Build history of the part. All positions in model axes, mm. A direction names the side the tool comes from. Coordinates: 2 decimals unless noted, no trailing zeros. Write each loop counter-clockwise with the first axis right and the second up, starting at its lowest first coordinate (ties: lowest second). Pieces come first, ordered by that corner, then holes. Notation, with made-up numbers: M 30,87.5 L 46,87.5 A27 cw 46,120.5 Z; hole C 59.5,-38.75 d4. An arc over 180 degrees is marked long. Use CSV: the item, a comma, the result in double quotes. Start each with the question number.
```python
from build123d import *

# Parameters (mm, degrees)
SKETCH1_R           = 2
BOSS_EXTRUDE1_DEPTH = 5
FILLET1_R           = 2


with BuildPart() as part:
    # Sketch1 → Boss-Extrude1 (new body)
    # profile 1 of 4: a face of its own
    with BuildSketch(Plane.XY):
        Polygon((8, 4), (-8, 4), (-8, 2.7), (-8, 0), (-8, -4), (8, -4), align=None)
        with Locations((-4, 0)):
            Circle(SKETCH1_R, mode=Mode.SUBTRACT)
        with BuildLine():
            ThreePointArc((6, 0), (4, -2), (2, 0))
            ThreePointArc((2, 0), (4, 2), (6, 0))
        make_face(mode=Mode.SUBTRACT)
    # profile 2 of 4: a face of its own
    with BuildSketch(Plane.XY):
        with BuildLine():
            Line((-8, 2.7), (-8, 4))
            Line((-8, 4), (-13.191868154, 4))
            ThreePointArc((-13.191868154, 4), (-13.048225449, 3.357041359), (-13, 2.7))
            Line((-13, 2.7), (-8, 2.7))
        make_face()
    # profile 3 of 4: a face of its own
    with BuildSketch(Plane.XY):
        with BuildLine():
            Line((-8, 0), (-8, 2.7))
            Line((-8, 2.7), (-13, 2.7))
            ThreePointArc((-13, 2.7), (-13.230925159, 1.276975053), (-13.9, 0))
            Line((-13.9, 0), (-8, 0))
        make_face()
    # profile 4 of 4: a face of its own
    with BuildSketch(Plane.XY):
        with BuildLine():
            ThreePointArc((-13, 2.7), (-13.048225449, 3.357041359), (-13.191868154, 4))
            ThreePointArc((-13.191868154, 4), (-21.931098884, 3.484450558), (-13.9, 0))
            ThreePointArc((-13.9, 0), (-13.230925159, 1.276975053), (-13, 2.7))
        make_face()
        with BuildLine():
            ThreePointArc((-20, 2.7), (-17.5, 5.2), (-15, 2.7))
            ThreePointArc((-15, 2.7), (-17.5, 0.2), (-20, 2.7))
        make_face(mode=Mode.SUBTRACT)
    extrude(amount=BOSS_EXTRUDE1_DEPTH)

    # Fillet1
    fillet1_edges = [part.edges().sort_by_distance(p)[0] for p in [
        (-8, 0, 2.5),
        (-13.9, 0, 2.5),
        (-13.191868154, 4, 2.5),
    ]]
    fillet(fillet1_edges, radius=FILLET1_R)


solid = part.part
```
1. Pull direction X, two halves, no side cores. Call faces 4 (the cylindrical face through (-13.764, -0.148, 2.535)), 5 (the flat face through (-7, 0, 0)), 6 (the flat face through (-8, -3, 2)): pulls with the +X half, pulls with the -X half, needs draft (parallel to the pull), parting line crosses it, or undercut.
2. Slice it at C-C (y = 2.7). List the corners of the cut face in (x, z), and give its area (3 significant figures).
3. 3-axis set-ups, long thin cutter, end or side, ignore diameter. For faces 1 (the flat face through (-2, 4, 2)), 2 (the cylindrical face through (-8.57, -0.6, 2.54)), 3 (the cylindrical face through (-21.933, 3.472, 2.465)): which of +Z, -Z, +X, -X, +Y, -Y reach the whole face in a straight line?
4. Slice it at D-D (y = 0.75). List the corners of the cut face in (x, z).
5. Slice it at B-B (z = 4.1). List the corners of the cut face in (x, y).
6. Drill centre lines: line 1 along Y through (x, z) = (4, 1.3); line 2 along Y through (x, z) = (-17.5, 1.2); line 3 along X through (y, z) = (-1.25, 3.55). Where is each one in solid material? Low to high. Write a range as from..to.
7. Slice it at A-A (x = 4). List the corners of the cut face in (y, z), and give its area (3 significant figures).
8. Flat gauge pins, fed straight in: pin 1 (3 mm diameter, centred on y = 0, z = 1, fed in from -X); pin 2 (1.5 mm diameter, centred on y = 3.5, z = 3, fed in from -X); pin 3 (2 mm diameter, centred on x = -12.5, z = 1.5, fed in from +Y); pin 4 (2.5 mm diameter, centred on x = -4, z = 3, fed in from +Y). Where does each tip first touch, or does it go through?
Established:
1,face 4,"undercut"
1,face 5,"needs draft"
1,face 6,"pulls with the -X half"
2,outline,"M -22,0 L -20,0 L -20,5 L -22,5 Z; M -15,0 L 8,0 L 8,5 L -15,5 Z"
2,area,"125 mm2"
3,face 1,"+Z, -Z, +X, +Y"
3,face 2,"+Z, -Z, -Y"
3,face 3,"+Z, -Z"
4,outline,"M -21.56,0 L -19.06,0 L -19.06,5 L -21.56,5 Z; M -15.94,0 L -5.85,0 L -5.85,5 L -15.94,5 Z; M -2.15,0 L 2.15,0 L 2.15,5 L -2.15,5 Z; M 5.85,0 L 8,0 L 8,5 L 5.85,5 Z"
5,outline,"M -14.39,-0.55 A2 cw -13.01,0 L -10,0 A2 cw -8,-2 L -8,-4 L 8,-4 L 8,4 L -11.9,4 A2 cw -13.62,4.98 A4.5 ccw long Z; hole C -17.5,2.7 d5; hole C -4,0 d4; hole C 4,0 d4"
6,line 1,"y = -4..-2, 2..4"
6,line 2,"y = -1.8..0.2, 5.2..7.2"
6,line 3,"x = -19.66..-15.34, -8.15..-5.56, -2.44..2.44, 5.56..8"
7,outline,"M -4,0 L -2,0 L -2,5 L -4,5 Z; M 2,0 L 4,0 L 4,5 L 2,5 Z"
7,area,"20.0 mm2"
8,pin 1,"stops at x = -21.84"
8,pin 2,"stops at x = -22"
8,pin 3,"stops at y = 4.8"
8,pin 4,"stops at y = 4"
